Autodesk Inventor part; units mm, degrees
ref_plane "YZ Plane" through (0, 0, 0) normal (1, 0, 0) x (0, 1, 0)
ref_plane "XZ Plane" through (0, 0, 0) normal (0, 1, 0) x (-1, 0, 0)
ref_plane "XY Plane" through (0, 0, 0) normal (0, 0, 1) x (1, 0, 0)
sketch "Boceto1" plane through (0, 0, 0) normal (0, 1, 0) x (-1, 0, 0)
  line L0 (16.15, 20) -> (-16.15, 20)
  line L1 (-16.15, 20) -> (-16.15, -20)
  line L2 (-16.15, -20) -> (16.15, -20)
  line L3 (16.15, -20) -> (16.15, 20)
  line L4 (0, -3.0912) -> (0, 0)
  line L5 (0, 0) -> (2.0406, 0)
  circle A0 centre (5.15, 13) radius 2
  circle A1 centre (5.15, -13) radius 2
  dimension "d0" = 32.3
  dimension "d1" = 40
  dimension "d4" = 4
  dimension "d5" = 4
  dimension "d6" = 7
  dimension "d7" = 7
  dimension "d35" = 11
  dimension "d36" = 11
extrude "Extrusión1" add sketch "Boceto1" along normal blind 5
sketch "Boceto2" plane through (0, 0, 0) normal (0, -1, 0) x (1, 0, 0)
  line L0 (16.15, 20) -> (16.15, -20)
  line L1 (16.15, 20) -> (11.15, 20)
  line L2 (11.15, 20) -> (11.15, -20)
  line L3 (11.15, -20) -> (16.15, -20)
  line L4 (16.15, -20) -> (16.15, 20)
  line L5 (-16.15, -20) -> (-16.15, 20)
  line L6 (-16.15, 20) -> (16.15, 20)
  line L7 (-16.15, -20) -> (-11.15, -20)
  line L8 (-11.15, -20) -> (-11.15, 20)
  line L9 (-11.15, 20) -> (-16.15, 20)
  line L10 (-16.15, 20) -> (-16.15, -20)
  point P0 (0, 0)
  dimension "d8" = 5
  dimension "d9" = 5
extrude "Extrusión2" add sketch "Boceto2" along normal blind 20
sketch "Boceto3" plane through (-11.15, 0, 20) normal (1, 0, 0) x (0, 0, -1)
  line L0 (0, 0) -> (0, -20)
  line L1 (40, -20) -> (40, 5)
  line L2 (0, -20) -> (40, -20)
  line L3 (40, -20) -> (40, -16)
  line L4 (40, -16) -> (0, -16)
  line L5 (0, -16) -> (0, -20)
  point P0 (20, 0)
  point P1 (0, -16)
  dimension "d12" = 4
extrude "Extrusión3" add sketch "Boceto3" along normal up to surface (22.3 mm away)
sketch "Boceto4" plane through (16.15, 5, 20) normal (1, 0, 0) x (0, 0, -1)
  circle A0 centre (21.15, -11.85) radius 2.5
  line L0 (0, 0) -> (0, -25)
  line L1 (0, 0) -> (40, 0)
  point P0 (20, -5)
  dimension "d15" = 21.15
  dimension "d16" = 11.85
  dimension "d19" = 5
extrude "Extrusión4" cut sketch "Boceto4" against normal up to surface (5 mm away)
sketch "Boceto8" plane through (0, -20, 0) normal (0, -1, 0) x (1, 0, 0)
  circle A0 centre (-5.15, 13) radius 2
  circle A1 centre (-5.15, -13) radius 2
  circle A2 centre (-5.15, 13) radius 2.5
  circle A3 centre (-5.15, -13) radius 2.5
  point P0 (0, 0)
  dimension "d31" = 5
  dimension "d32" = 5
extrude "Extrusión7" cut sketch "Boceto8" against normal up to surface (4 mm away) contours A0 | A1 | A2 | A3
sketch "Boceto9" plane through (0, 0, 0) normal (0, -1, 0) x (1, 0, 0)
  line L0 (-16.15, -20) -> (-16.15, 20)
  line L1 (-16.15, 5) -> (-1.15, 5)
  line L2 (-1.15, 5) -> (-1.15, -5)
  line L3 (-1.15, -5) -> (-16.15, -5)
  line L4 (-16.15, -5) -> (-16.15, 5)
  line L5 (-18.3593, 0) -> (-23.2163, 0)
  point P0 (0, 0)
  dimension "d37" = 15
  dimension "d38" = 10
extrude "Extrusión8" add sketch "Boceto9" along normal up to surface (20 mm away)
sketch "Boceto5" plane through (-16.15, 5, -20) normal (-1, 0, 0) x (0, 0, 1)
  circle A0 centre (18.85, -11.85) radius 2.5
  point P0 (20, -5)
hole "Agujero1" at (-16.15, -6.85, -1.15) direction (1, 0, 0) diameter 7 depth 15
sketch "Boceto10" plane through (-1.15, 0, 5) normal (1, 0, 0) x (0, 0, -1)
  circle A0 centre (6.15, -6.85) radius 3.5
  circle A1 centre (6.15, -6.85) radius 2.5
  point P0 (5, 0)
  dimension "d41" = 5
extrude "Extrusión9" add sketch "Boceto10" against normal blind 5
sketch "Boceto11" plane through (-16.15, 5, 20) normal (0, 0, 1) x (1, 0, 0)
  point P0 (16.15, -5)
sketch "Boceto12" plane through (-16.15, 5, 20) normal (0, 0, 1) x (1, 0, 0)
  line L0 (5, -5) -> (27.3, -5)
  line L1 (27.3, -5) -> (15, -5)
  line L2 (15, -5) -> (15, -3)
  line L3 (15, -3) -> (27.3, -3)
  line L4 (27.3, -3) -> (27.3, -5)
  point P0 (16.15, -5)
  dimension "d44" = 2
extrude "Extrusión10" cut sketch "Boceto12" against normal up to surface (40 mm away)
chamfer "Chaflán1" distance 1 angle 45 1 edges at (-1.15, -6.85, 1.35)
sketch "Boceto13" plane through (16.15, 5, 20) normal (1, 0, 0) x (0, 0, -1)
  line L0 (40, -25) -> (40, 0)
  line L1 (40, 0) -> (22, 0)
  line L2 (22, 0) -> (22, -5)
  line L3 (22, -5) -> (40, -5)
  line L4 (40, -5) -> (40, 0)
  point P0 (20, -5)
  dimension "d50" = 18
  dimension "d51" = 5
extrude "Extrusión11" cut sketch "Boceto13" against normal blind 10
sketch "Boceto16" plane through (16.15, -20, 20) normal (1, 0, 0) x (0, 0, -1)
  circle A0 centre (4, 21) radius 2
  circle A1 centre (14, 21) radius 2
  line L0 (0, 25) -> (0, 0)
  line L1 (0, 25) -> (22, 25)
  point P0 (20, 20)
  dimension "d66" = 4
  dimension "d67" = 4
  dimension "d68" = 10
  dimension "d69" = 4
  dimension "d70" = 4
  dimension "d71" = 4
extrude "Extrusión14" cut sketch "Boceto16" against normal blind 5
equation "\"d5\" = d4"
equation "\"d36\" = d35"
equation "\"d9\" = d8"
equation "\"d67\" = d66"
equation "\"d71\" = d70"
properties part number "Base Idler Izq" material "Plástico PAEK"
Model file for the job. Use its own axes, mm. A direction names the side the tool comes from. Coordinates: 2 decimals unless noted, no trailing zeros. Write each loop counter-clockwise with the first axis right and the second up, starting at its lowest first coordinate (ties: lowest second). Pieces come first, ordered by that corner, then holes. Notation, with made-up numbers: (69, -0.5) - (87, -0.5) arc R13 cw to (87, 4.5) - close; hole circle Ø11 at (39, 16.5). An arc over 180 degrees is marked (long way). One line per question, with ' | ' between items. Start each with the question number.
Q1. Pin check, flat tips, straight feed: pin 1 (3.5 mm diameter, centred on y = -7.5, z = -2.5, fed in from -X); pin 2 (3 mm diameter, centred on x = -6.5, y = -7.5, fed in from -Z); pin 3 (3.5 mm diameter, centred on y = 3.5, z = -7, fed in from +X). Stop position of each tip, or through.
Q2. Cut at D-D, the plane z = -1.15. List the corners of the cut face in (x, y).
Q3. 3-axis set-ups, long thin cutter, end or side, ignore diameter. For faces 4 (the face through (-6, -8, -5)), 5 (the face through (-5.69, -18.03, -15.44)), 6 (the face through (-6, -8, 5)): which of +Z, -Z, +X, -X, +Y, -Y reach the whole face in a straight line?
Q4. Cut at B-B, the plane z = -13. List the corners of the cut face in (x, y), then the cut area to 3 significant figures.
Q5. Cut at C-C, the plane y = -2. List the corners of the cut face in (x, z).
Q6. Pull direction Y, two halves, no side cores. Call faces 1 (the face through (0, 5, 0)), 2 (the face through (16.15, -10, 0)), 3 (the face through (13.7, -0.2, 17.6)): pulls with the +Y half, pulls with the -Y half, needs draft (parallel to the pull), parting line crosses it, or undercut.
Q7. Drill centre lines: line 1 (Z direction, x = -5.15, y = 2.6); line 2 (X direction, y = -11.5, z = 4); line 3 (X direction, y = -2.5, z = 15.5). Where is each one in solid material? Low to high. Write a range as [from, to].
Q8. Cut at A-A, the plane x = -5.15. Give the number of separate pieces and of enclosed holes in the cut face, then the cut area to 3 significant figures.
Answer below:
1) pin 1: x = -6.15 | pin 2: z = -5 | pin 3: x = 6.15
2) outline: (-16.15, -20) - (16.15, -20) - (16.15, -9.35) - (11.15, -9.35) - (11.15, -16) - (-1.15, -16) - (-1.15, -10.35) - (-2.15, -9.35) - (-6.15, -9.35) - (-6.15, -10.35) - (-16.15, -10.35) - close; (-16.15, -3.35) - (-6.15, -3.35) - (-6.15, -4.35) - (-2.15, -4.35) - (-1.15, -3.35) - (-1.15, 2) - (11.15, 2) - (11.15, -4.35) - (16.15, -4.35) - (16.15, 5) - (-16.15, 5) - close
3) face 4: -Z | face 5: -Y | face 6: +Z
4) outline: (-16.15, -20) - (-7.65, -20) - (-7.65, -16) - (-11.15, -16) - (-11.15, 0) - (-7.15, 0) - (-7.15, 5) - (-16.15, 5) - close; (-3.15, 0) - (-1.15, 0) - (-1.15, 2) - (6.15, 2) - (6.15, 5) - (-3.15, 5) - close; (-2.65, -20) - (16.15, -20) - (16.15, 0) - (11.15, 0) - (11.15, -16) - (-2.65, -16) - close | area: 346 mm^2
5) outline: (-16.15, -20) - (-11.15, -20) - (-11.15, -5) - (-1.15, -5) - (-1.15, 5) - (-11.15, 5) - (-11.15, 20) - (-16.15, 20) - close; (11.15, -20) - (16.15, -20) - (16.15, 20) - (11.15, 20) - close
6) face 1: pulls with the +Y half | face 2: needs draft | face 3: undercut
7) line 1: [-20, -15], [-11, 11], [15, 20] | line 2: [-16.15, -1.15], [11.15, 16.15] | line 3: [-16.15, -11.15], [11.15, 16.15]
8) separate pieces: 5 | enclosed holes: 1 | area: 420 mm^2
